The listing builds one solid part. Answer for the finished solid, in the listing's coordinates (mm). A direction names the side the tool comes from. Coordinates: 2 decimals unless noted, no trailing zeros. Order: outer loops, then holes, each group sorted by start corner. A loop starts at its lowest first (then second) coordinate and runs counter-clockwise, first axis right, second up. Notation, with made-up numbers: (-20, 5) -> (27, 5) arc R13 cw to (27, 24) -> close; hole circle Ø10 at (58.5, 26). An arc over 180 degrees is marked (long way). One line per question, with ' | ' between items.
Autodesk Inventor part; units mm, degrees
ref_plane "YZ Plane" through (0, 0, 0) normal (1, 0, 0) x (0, 1, 0)
ref_plane "XZ Plane" through (0, 0, 0) normal (0, 1, 0) x (-1, 0, 0)
ref_plane "XY Plane" through (0, 0, 0) normal (0, 0, 1) x (1, 0, 0)
sketch "Sketch1" plane through (0, 0, 0) normal (0, 1, 0) x (-1, 0, 0)
  line L0 (7.0481, 13.5339) -> (-297.7519, 13.5339)
  line L1 (-297.7519, 13.5339) -> (-297.7519, -291.2661)
  line L2 (-297.7519, -291.2661) -> (7.0481, -291.2661)
  line L3 (7.0481, -291.2661) -> (7.0481, 13.5339)
  arc A0 (-297.7519, 13.5339) -> (-297.7519, -291.2661) centre (83.7145, -138.8661) ccw
  point P0 (0, 0)
  dimension "d0" = 304.8
  dimension "d1" = 304.8
extrude "Extrusion1" add sketch "Sketch1" along normal blind 25.4
sketch "Sketch2" plane through (0, 25.4, 0) normal (0, 1, 0) x (1, 0, 0)
  line L0 (-7.0481, 291.2661) -> (-7.0481, -13.5339)
  line L1 (-7.0481, 138.8661) -> (145.3519, 138.8661)
  circle A0 centre (145.3519, 138.8661) radius 19.05
  point P0 (0, 0)
  dimension "d4" = 152.4
  dimension "d5" = 38.1
extrude "Extrusion2" cut sketch "Sketch2" against normal blind 50.8
sketch "Sketch3" plane through (0, 25.4, 0) normal (0, 1, 0) x (1, 0, 0)
  line L0 (-7.0481, 291.2661) -> (-7.0481, -13.5339)
  line L1 (297.7519, 291.2661) -> (-7.0481, 291.2661)
  line L2 (-7.0481, -13.5339) -> (297.7519, 291.2661)
  line L3 (-7.0481, -13.5339) -> (297.7519, -13.5339)
  line L4 (-7.0481, 291.2661) -> (297.7519, -13.5339)
  line L5 (-7.0481, -13.5339) -> (28.873, 22.3871)
  line L6 (297.7519, -13.5339) -> (261.8309, 22.3871)
  line L7 (297.7519, 291.2661) -> (261.8309, 255.3451)
  line L8 (-7.0481, 291.2661) -> (28.873, 255.3451)
  line L9 (28.873, 22.3871) -> (261.8309, 22.3871)
  line L10 (261.8309, 22.3871) -> (261.8309, 255.3451)
  line L11 (261.8309, 255.3451) -> (28.873, 255.3451)
  line L12 (28.873, 255.3451) -> (28.873, 22.3871)
  line L13 (28.873, 22.3871) -> (100.715, 94.2292) construction
  line L14 (37.8532, 13.4068) -> (109.6953, 85.2489)
  line L15 (91.7348, 103.2094) -> (19.8927, 31.3674)
  arc A0 (19.8927, 31.3674) -> (37.8532, 13.4068) centre (28.873, 22.3871) ccw
  arc A1 (109.6953, 85.2489) -> (91.7348, 103.2094) centre (100.715, 94.2292) ccw
  line L16 (28.873, 255.3451) -> (100.715, 183.503) construction
  line L17 (19.8927, 246.3648) -> (91.7348, 174.5228)
  line L18 (109.6953, 192.4833) -> (37.8532, 264.3253)
  arc A2 (37.8532, 264.3253) -> (19.8927, 246.3648) centre (28.873, 255.3451) ccw
  arc A3 (91.7348, 174.5228) -> (109.6953, 192.4833) centre (100.715, 183.503) ccw
  line L19 (261.8309, 22.3871) -> (189.9889, 94.2292) construction
  line L20 (270.8112, 31.3674) -> (198.9691, 103.2094)
  line L21 (181.0086, 85.2489) -> (252.8507, 13.4068)
  arc A4 (252.8507, 13.4068) -> (270.8112, 31.3674) centre (261.8309, 22.3871) ccw
  arc A5 (198.9691, 103.2094) -> (181.0086, 85.2489) centre (189.9889, 94.2292) ccw
  line L22 (261.8309, 255.3451) -> (189.9889, 183.503) construction
  line L23 (252.8507, 264.3253) -> (181.0086, 192.4833)
  line L24 (198.9691, 174.5228) -> (270.8112, 246.3648)
  arc A6 (270.8112, 246.3648) -> (252.8507, 264.3253) centre (261.8309, 255.3451) ccw
  arc A7 (181.0086, 192.4833) -> (198.9691, 174.5228) centre (189.9889, 183.503) ccw
  point P0 (0, 0)
  point P1 (64.794, 58.3081)
  point P2 (64.794, 219.424)
  point P3 (225.9099, 58.3081)
  point P4 (225.9099, 219.424)
  dimension "d8" = 50.8
  dimension "d9" = 50.8
  dimension "d10" = 50.8
  dimension "d11" = 50.8
  dimension "d12" = 101.6
  dimension "d13" = 25.4
  dimension "d14" = 101.6
  dimension "d15" = 25.4
  dimension "d16" = 101.6
  dimension "d17" = 25.4
  dimension "d18" = 101.6
  dimension "d19" = 25.4
extrude "Extrusion3" cut sketch "Sketch3" against normal blind 50.8 contours A2 L18 L11 L4 | L4 L12 L17 A2 | A0 L15 L12 L2 | L2 L9 L14 A0 | A6 L24 L10 L2 | L2 L11 L23 A6 | L11 L18 A3 L4 | L4 A3 L17 L12 | L12 L15 A1 L2 | L2 A1 L14 L9 | A4 L21 L9 L4 | L4 L10 L20 A4 | L10 L24 A7 L2 | L2 A7 L23 L11 | L9 L21 A5 L4 | L4 A5 L20 L10
properties part number "Shoddy Drilling Platform Representation"
Item 1: Each of these flat-tipped pins is pushed along its axis until it touches: pin 1 Ø5 at (y, z) = (7.5, -25) entering from +X; pin 2 Ø2 at (x, z) = (213.5, -225) entering from -Y. Where does it stop, or does it pass through?
Computed values:
pin 1: stops at x = 311.68 | pin 2: stops at y = 0
Item 2: Section A-A, the plane x = 217 is taken. Give the vertices of the cut face in (y, z), plus the area to 3 significant figures.
Computed values:
outline: (0, -291.27) -> (25.4, -291.27) -> (25.4, -228.47) -> (0, -228.47) -> close; (0, -192.55) -> (25.4, -192.55) -> (25.4, -85.18) -> (0, -85.18) -> close; (0, -49.26) -> (25.4, -49.26) -> (25.4, 13.53) -> (0, 13.53) -> close | area: 5,920 mm^2
Item 3: Section B-B, the plane z = -226.5 is taken. Give the vertices of the cut face in (x, y).
Computed values:
outline: (-7.05, 0) -> (39.76, 0) -> (39.76, 25.4) -> (-7.05, 25.4) -> close; (75.68, 0) -> (215.03, 0) -> (215.03, 25.4) -> (75.68, 25.4) -> close; (250.95, 0) -> (317.61, 0) -> (317.61, 25.4) -> (250.95, 25.4) -> close
Item 4: For faces 1 (the face through (234.387, 12.878, -209.941)), 2 (the face through (143, 13, 13.534)), determine the directions among +Z, -Z, +X, -X, +Y, -Y from which every point of the face is accessible in a straight line to the end or side of a thin tool.
Computed values:
face 1: +Y, -Y | face 2: +Z, +X, -X, +Y, -Y
Item 5: Find the intervals of material crossed by L1, parallel to X at y = 10, z = -49.5; L2, parallel to Z at x = 273, y = 10.25; L3, parallel to X at y = 4, z = -57.5, in increasing order.
Computed values:
L1: x = -7.05 to 38.03, 73.95 to 216.76, 252.68 to 317.23 | L2: z = -291.27 to -261.39, -249.3 to -28.43, -16.34 to 13.53 | L3: x = -7.05 to 46.03, 81.95 to 208.76, 244.68 to 318.93
Item 6: Section D-D, the plane y = 5.5 is taken. Count the separate pieces of the cut face and the enclosed holes in it, plus the area to 3 significant figures.
Computed values:
separate pieces: 1 | enclosed holes: 5 | area: 85,400 mm^2
Item 7: Section C-C, the plane x = 156 is taken. Give the vertices of the cut face in (y, z).
Computed values:
outline: (0, -291.27) -> (25.4, -291.27) -> (25.4, -154.66) -> (0, -154.66) -> close; (0, -123.07) -> (25.4, -123.07) -> (25.4, 13.53) -> (0, 13.53) -> close
Item 8: Determine the mould class of faces 3 (the face through (-7.048, 13, -141)), 4 (the face through (147, 13, -291.266)), 5 (the face through (217.433, 12.878, -228.907)) for opening direction Z: pulls with the +Z half, pulls with the -Z half, needs draft (parallel to the pull), parting line crosses it, or undercut.
Computed values:
face 3: needs draft | face 4: pulls with the -Z half | face 5: undercut
